Input: part model. Units: mm. Frame: model coordinates. A direction names the side the tool comes from. Round coordinates to 2 decimals unless told otherwise and drop trailing zeros. Loops run counter-clockwise (first coordinate to the right, second up) from the corner with the lowest first, then second, coordinate; pieces in that order, holes last.
(1) Cut plane C-C, the plane x = 10.2. Output: boundary loops of the cut face in (y, z), and give its area (4 significant figures).
(2) Line query: line 1 (X direction, y = -15.9, z = 12.5); line 2 (Y direction, x = -8.25, z = 1); line 3 (Z direction, x = -10.2, y = -0.35). Output: solid intervals per line, ascending.
(3) Cut plane A-A, the plane y = -1. Output: boundary loops of the cut face in (x, z).
(4) Access query for faces 1 (the face through (-12.7, -1, 0)), 2 (the face through (-2, -11, 0)), 3 (the face through (9, -1, 0)), 4 (the face through (11.415, -1.5, 0.591)), 5 (the face through (0, -15.5, 6)). Directions: +Z, -Z, +X, -X, +Y, -Y. A direction counts if a zero-diameter tool reaches every point of the face in a straight line with its end or side. Return the directions, or none.
(5) Cut plane B-B, the plane z = 0. Give the number of separate pieces and of enclosed holes in the cut face, and give its area (3 significant figures).
(6) First-contact query: pin 1 Ø1.5 at (y, z) = (-11.5, 0.5) entering from +X; pin 2 Ø6 at (x, z) = (8.5, 13) entering from +Y; pin 3 Ø1.5 at (y, z) = (-10, -1) entering from -X. Flat tips, straight axial feed; report the tip coordinate or a pass-through.
(7) Draft query along X for faces 6 (the face through (0.049, -15.238, 3.153)), 7 (the face through (-5.078, -4.818, 0.035)), 8 (the face through (-0.1, -5.5, 0)). Return one class per face: released by +X, released by -X, zero draft, split by the parting line, or undercut.
(8) Cut plane D-D, the plane x = 7. Output: boundary loops of the cut face in (y, z).
from build123d import *

# Parameters (mm, degrees)
BOSS_EXTRUDE1_DEPTH = 2.5
SKETCH2_R           = 1.2
CUT_EXTRUDE1_DEPTH  = 8
BOSS_EXTRUDE2_START = -15.5
SKETCH3_W           = 4
SKETCH3_H           = 5
BOSS_EXTRUDE2_DEPTH = 8.791796
SKETCH4_W           = 25.4
SKETCH4_H           = 17.5
BOSS_EXTRUDE3_DEPTH = 1.5
FILLET1_R           = 1.5
SKETCH5_R           = 1.2
CUT_EXTRUDE2_DEPTH  = 18


with BuildPart() as part:
    # Sketch1 → Boss-Extrude1 (new body, symmetric)
    with BuildSketch(Plane.XY):
        with BuildLine():
            Line((5.5, 0), (12.7, 0))
            Line((12.7, 0), (12.7, -1.5))
            Line((12.7, -1.5), (6.837397166, -1.5))
            ThreePointArc((6.837397166, -1.5), (0, -7), (-6.837397166, -1.5))
            Line((-6.837397166, -1.5), (-12.7, -1.5))
            Line((-12.7, -1.5), (-12.7, 0))
            Line((-12.7, 0), (-5.5, 0))
            ThreePointArc((-5.5, 0), (0, -5.5), (5.5, 0))
        make_face()
    extrude(amount=BOSS_EXTRUDE1_DEPTH, both=True)

    # Sketch2 → Cut-Extrude1 (cut, through all)
    with BuildSketch(Plane(origin=(0, 0, 0), x_dir=(1, 0, 0), z_dir=(0, 1, 0))):
        with Locations((-10.2, 0)):
            Circle(SKETCH2_R)
        with Locations((10.2, 0)):
            Circle(SKETCH2_R)
    extrude(amount=-CUT_EXTRUDE1_DEPTH, mode=Mode.SUBTRACT)

    # Sketch3 → Boss-Extrude2 (add)
    with BuildSketch(Plane(origin=(0, 0, 0), x_dir=(1, 0, 0), z_dir=(0, 1, 0)).offset(BOSS_EXTRUDE2_START)):
        Rectangle(SKETCH3_W, SKETCH3_H)
    extrude(amount=BOSS_EXTRUDE2_DEPTH)

    # Sketch4 → Boss-Extrude3 (add)
    with BuildSketch(Plane.XZ.offset(15.5)):
        with Locations((0, 6.25)):
            Rectangle(SKETCH4_W, SKETCH4_H)
    extrude(amount=BOSS_EXTRUDE3_DEPTH)

    # Fillet1
    fillet1_edges = [part.edges().sort_by_distance(p)[0] for p in [
        (6.837397166, -1.5, 0),
        (-6.837397166, -1.5, 0),
        (2, -15.5, 0),
        (-2, -15.5, 0),
        (0, -15.5, 2.5),
        (2, -6.708204, 0),
        (-2, -6.708204, 0),
    ]]
    fillet(fillet1_edges, radius=FILLET1_R)

    # Sketch5 → Cut-Extrude2 (cut, through all)
    with BuildSketch(Plane(origin=(0, 0, 0), x_dir=(1, 0, 0), z_dir=(0, 1, 0))):
        with Locations((-5, -12.5)):
            Circle(SKETCH5_R)
        with Locations((5, -12.5)):
            Circle(SKETCH5_R)
    extrude(amount=-CUT_EXTRUDE2_DEPTH, mode=Mode.SUBTRACT)


solid = part.part
Reported:
1. outline: (-17, -2.5) - (-15.5, -2.5) - (-15.5, 15) - (-17, 15) - close; (-1.5, -2.5) - (0, -2.5) - (0, -1.2) - (-1.5, -1.2) - close; (-1.5, 1.2) - (0, 1.2) - (0, 2.5) - (-1.5, 2.5) - close
1. area: 30.15 mm2
2. line 1: x = -12.7 to -6.2, -3.8 to 3.8, 6.2 to 12.7
2. line 2: y = -17 to -15.5, -1.5 to 0
2. line 3: z = -2.5 to -1.2, 1.2 to 2.5
3. outline: (-12.7, -2.5) - (-5.41, -2.5) - (-5.41, 2.5) - (-12.7, 2.5) - close; (5.41, -2.5) - (12.7, -2.5) - (12.7, 2.5) - (5.41, 2.5) - close; hole circle Ø2.4 at (-10.2, 0); hole circle Ø2.4 at (10.2, 0)
4. face 1: +Z, -Z, -X, +Y, -Y
4. face 2: +Z, -Z, -X
4. face 3: +Y
4. face 4: +Z, -Z, +X
4. face 5: +Z
5. separate pieces: 3
5. enclosed holes: 0
5. area: 114 mm2
6. pin 1: stops at x = 2
6. pin 2: stops at y = -15.5
6. pin 3: stops at x = -2
7. face 6: zero draft
7. face 7: released by -X
7. face 8: undercut
8. outline: (-17, -2.5) - (-15.5, -2.5) - (-15.5, 15) - (-17, 15) - close; (-1.84, -2.5) - (0, -2.5) - (0, 2.5) - (-1.84, 2.5) - close
